```python
from build123d import *

# Parameters (mm, degrees)
EXTRUDE_1_DEPTH = 10
FILLET_7_R      = 20


with BuildPart() as part:
    # 草图1 → 凸台-拉伸1 (new body)
    with BuildSketch(Plane(origin=(0, 0, 0), x_dir=(1, 0, 0), z_dir=(0, 1, 0))):
        Polygon((-120, 32.5), (120, 32.5), (120, 212.5), (150, 212.5), (150, 32.5), (150, -32.5), (-150, -32.5), (-150, 32.5), (-150, 212.5), (-120, 212.5), align=None)
    extrude(amount=EXTRUDE_1_DEPTH)

    # 圆角7
    fillet_7_edges = [part.edges().sort_by_distance(p)[0] for p in [
        (-120, 5, -32.5),
        (120, 5, -32.5),
    ]]
    fillet(fillet_7_edges, radius=FILLET_7_R)


solid = part.part
```
Input: part model. Units: mm. Frame: model coordinates. A direction names the side the tool comes from. Round coordinates to 2 decimals unless told otherwise and drop trailing zeros. Loops run counter-clockwise (first coordinate to the right, second up) from the corner with the lowest first, then second, coordinate; pieces in that order, holes last.
1) Set-up query: faces 4 (the cylindrical face through (-113.986, 5.07, -38.203)), 5 (the flat face through (2, 10, -10)). Return all of +Z, -Z, +X, -X, +Y, -Y with unobstructed straight access to the full face (end or side cutting, diameter ignored); none if empty.
Ans:
face 4: -Z, +Y, -Y
face 5: +Z, -Z, +X, -X, +Y
2) Section query D-D on x = -68.5. Return the cut outline in (y, z).
Ans:
outline: (0, -32.5) - (10, -32.5) - (10, 32.5) - (0, 32.5) - close
3) Material intervals for line 1 (X direction, y = 1.25, z = -66.5); line 2 (Z direction, x = -82, y = 4); line 3 (Z direction, x = 105, y = 5.75), sorted ascending.
Ans:
line 1: x = -150 to -120, 120 to 150
line 2: z = -32.5 to 32.5
line 3: z = -33.14 to 32.5
4) Section query A-A on z = -159.5. Return the cut outline in (x, y).
Ans:
outline: (-150, 0) - (-120, 0) - (-120, 10) - (-150, 10) - close; (120, 0) - (150, 0) - (150, 10) - (120, 10) - close
5) Section query C-C on z = -47. Return the cut outline in (x, y).
Ans:
outline: (-150, 0) - (-119.23, 0) - (-119.23, 10) - (-150, 10) - close; (119.23, 0) - (150, 0) - (150, 10) - (119.23, 10) - close
6) Pull-direction query (X, two-part tool) for faces 1 (the flat face through (-150, 5, -92)), 2 (the flat face through (2, 0, -10)), 3 (the flat face through (120, 5, -131)); classes: released by +X, released by -X, zero draft, split by the parting line, or undercut.
Ans:
face 1: released by -X
face 2: zero draft
face 3: undercut
7) Pin query (flat end, axial travel): pin 1 (5 mm diameter, centred on x = 48.5, y = 3.5, fed in from -Z); pin 2 (2 mm diameter, centred on x = -103.5, y = 6.5, fed in from -Z); pin 3 (1.5 mm diameter, centred on x = 28, z = -5.5, fed in from -Y). Return the tip coordinate at first contact, or that it passes through.
Ans:
pin 1: stops at z = -32.5
pin 2: stops at z = -33.01
pin 3: stops at y = 0
8) Section query B-B on y = 7.5. Return the cut outline in (x, z), plus the area to 3 significant figures.
Ans:
outline: (-150, -212.5) - (-120, -212.5) - (-120, -52.5) arc R20 cw to (-100, -32.5) - (100, -32.5) arc R20 cw to (120, -52.5) - (120, -212.5) - (150, -212.5) - (150, 32.5) - (-150, 32.5) - close
area: 30,500 mm2
